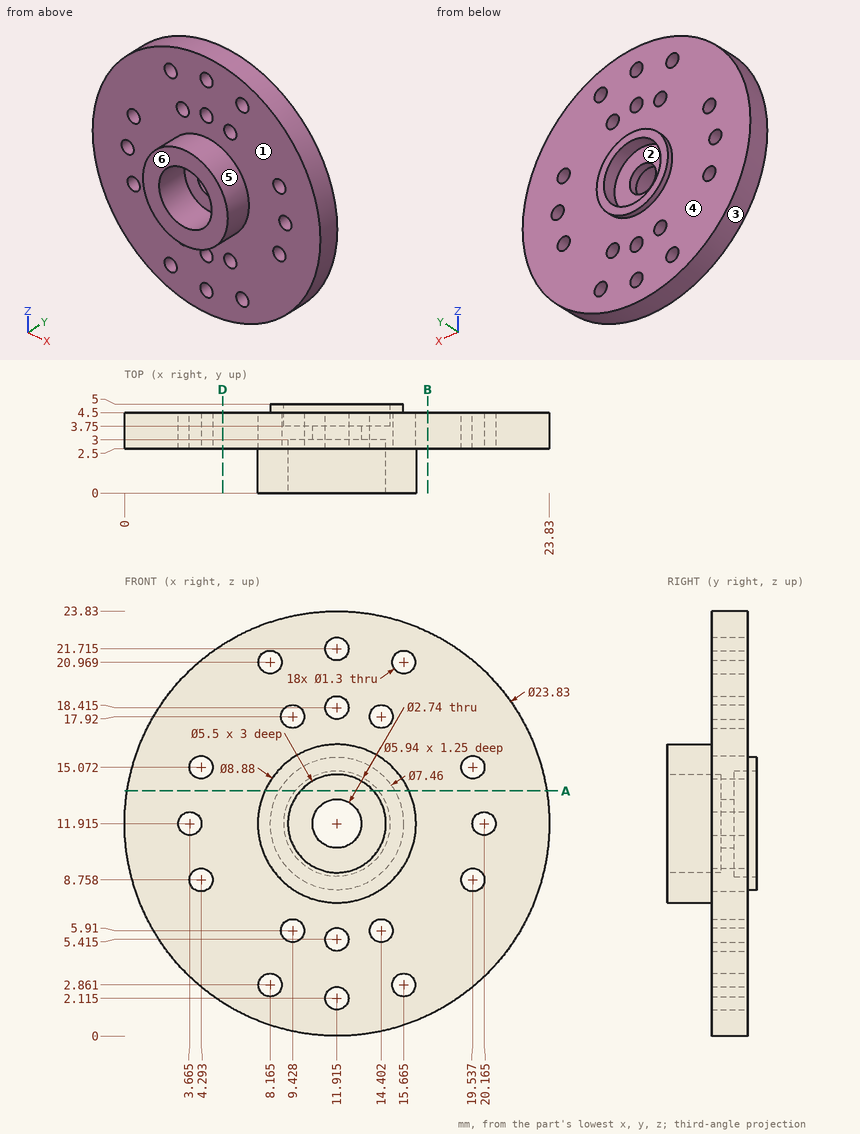
Design review of the part shown in the three views and the two pictorial views. Dimensions are in mm from the part's minimum x, y and z. A direction names the side the tool comes from. Coordinates: 2 decimals unless noted, no trailing zeros. Order: outer loops, then holes, each group sorted by start corner. A loop starts at its lowest first (then second) coordinate and runs counter-clockwise, first axis right, second up.
1) Mouldability with a two-part tool opening along Z and no side actions: class the marked faces 1, 2 and 3 as +Z half, -Z half, draft (parallel to the pull), parting line (faces both ways), or undercut.
2) Wall thickness on line 1 along X through (y, z) = (3.75, 21) (1 decimal); line 2 along X through (y, z) = (3.6, 17.5) (1 decimal); line 3 along Y through (x, z) = (19, 9.25): over which ranges is each line inside the solid? List them lowest first.
3) For the marked faces 4, 5 and 6, list the 3-axis set-ups (+Z, -Z, +X, -X, +Y, -Y) from which the entire face can be reached by the end or side of a thin tool; tool diameter is ignored.
4) Take a section at D-D, the plane x = 5.5. Give the boundary of the cut face in (y, z) (1 decimal).
5) Take a section at A-A, the plane z = 13.75. Give the boundary of the cut face in (x, y).
6) Take a section at B-B, the plane x = 17. Give the boundary of the cut face in (y, z).
7) Clearance check with flat-ended pins moving along their axes: pin 1 (1.5 mm diameter, centred on x = 11.915, z = 2.115, fed in from +Y); pin 2 (1 mm diameter, centred on x = 2.5, y = 2.5, fed in from -Z); pin 3 (2 mm diameter, centred on x = 11.915, z = 21.715, fed in from -Y). State where each tip first meets the part, or that it passes through.
Returned:
1. face 1: draft
1. face 2: undercut
1. face 3: parting line
2. line 1: x = 4.2 to 7.5, 8.8 to 15, 16.3 to 19.6
2. line 2: x = 1.4 to 8.9, 9.9 to 13.9, 14.9 to 22.4
2. line 3: y = 2.5 to 4.5
3. face 4: +Y
3. face 5: -Y
3. face 6: +Z, -Z, +X, -X, -Y
4. outline: (2.5, 1.9) - (4.5, 1.9) - (4.5, 22) - (2.5, 22) - close
5. outline: (0.14, 2.5) - (7.87, 2.5) - (7.87, 0) - (9.87, 0) - (9.87, 3) - (13.96, 3) - (13.96, 0) - (15.96, 0) - (15.96, 2.5) - (23.69, 2.5) - (23.69, 4.5) - (15.16, 4.5) - (15.16, 5) - (14.25, 5) - (14.25, 3.75) - (9.58, 3.75) - (9.58, 5) - (8.67, 5) - (8.67, 4.5) - (0.14, 4.5) - close
6. outline: (2.5, 1.14) - (4.5, 1.14) - (4.5, 22.69) - (2.5, 22.69) - close
7. pin 1: stops at y = 4.5
7. pin 2: stops at z = 4.01
7. pin 3: stops at y = 2.5
